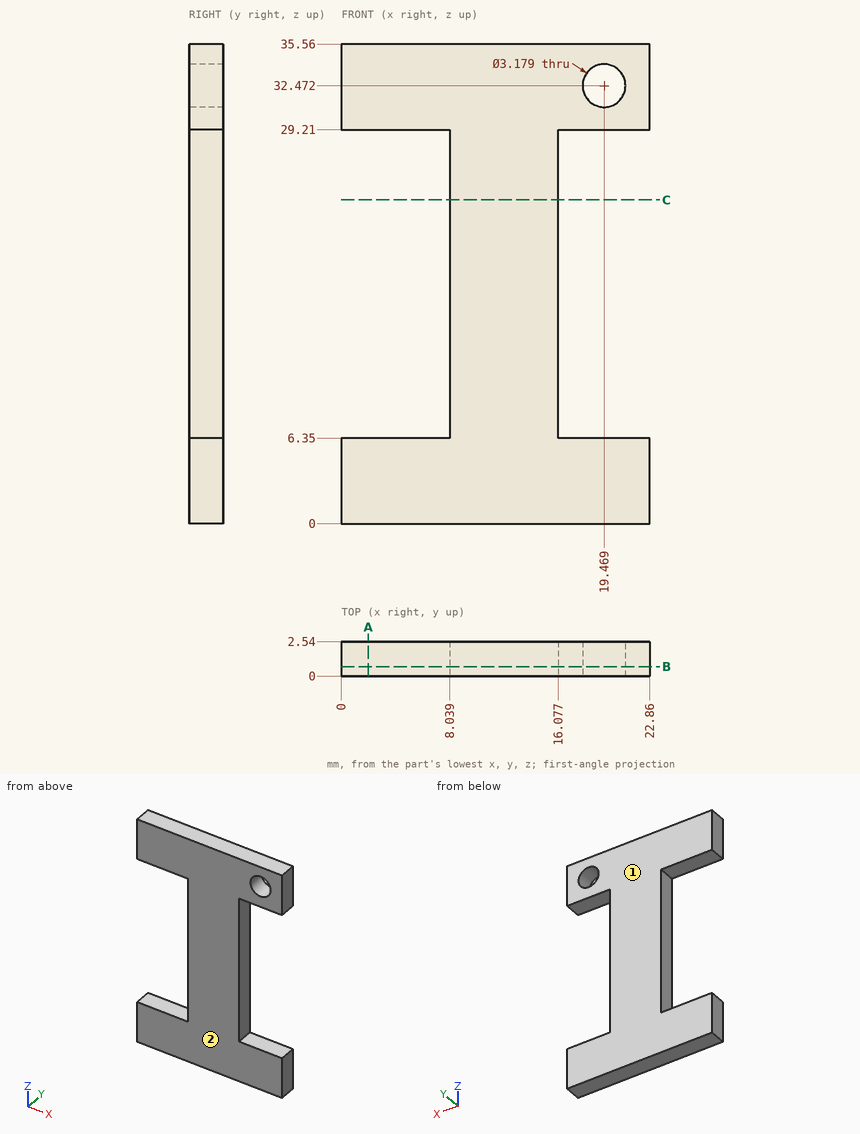
Input: dimensioned drawing with shaded views. Units: mm. Origin: part minimum x, y, z. Round coordinates to 2 decimals unless told otherwise and drop trailing zeros. Loops run counter-clockwise (first coordinate to the right, second up) from the corner with the lowest first, then second, coordinate; pieces in that order, holes last. Notation, with made-up numbers: M -38,47 L -31,47 A19 ccw -31,82 Z; hole C 37.25,-28.5 d8. An arc over 180 degrees is marked long. Return JSON: item names as keys, results as strings. Group by question number.
1. Material intervals for line 1 along Z through (x, y) = (2.75, 0.95); line 2 along Z through (x, y) = (20, 1.65); line 3 along X through (y, z) = (2.05, 9.5), sorted ascending. Write a range as from..to.
2. Section query C-C on z = 24. Output: boundary loops of the cut face in (x, y).
3. Pin query (flat end, axial travel): pin 1 (1.5 mm diameter, centred on y = 2, z = 12, fed in from +X); pin 2 (4 mm diameter, centred on x = 5.5, z = 19, fed in from +Y). Return the tip coordinate at first contact, or that it passes through.
4. Section query A-A on x = 2. Output: boundary loops of the cut face in (y, z).
5. Section query B-B on y = 0.7. Output: boundary loops of the cut face in (x, z).
6. Mould query, pull axis Y, two halves, no side actions, for the marked faces 1 and 2. Classes: released by +Y, released by -Y, zero draft, split by the parting line, or undercut.
Checks:
{
 "1": {"line 1": "z = 0..6.35, 29.21..35.56", "line 2": "z = 0..6.35, 29.21..30.97, 33.97..35.56", "line 3": "x = 8.04..16.08"},
 "2": {"outline": "M 8.04,0 L 16.08,0 L 16.08,2.54 L 8.04,2.54 Z"},
 "3": {"pin 1": "stops at x = 16.08", "pin 2": "passes through"},
 "4": {"outline": "M 0,0 L 2.54,0 L 2.54,6.35 L 0,6.35 Z; M 0,29.21 L 2.54,29.21 L 2.54,35.56 L 0,35.56 Z"},
 "5": {"outline": "M 0,0 L 22.86,0 L 22.86,6.35 L 16.08,6.35 L 16.08,29.21 L 22.86,29.21 L 22.86,35.56 L 0,35.56 L 0,29.21 L 8.04,29.21 L 8.04,6.35 L 0,6.35 Z; hole C 19.47,32.47 d3.18"},
 "6": {"face 1": "released by +Y", "face 2": "released by -Y"}
}
